Here's how the part is built. I have some questions about the finished solid (model axes, mm). A direction names the side the tool comes from. Round coordinates to 2 decimals unless told otherwise and drop trailing zeros. Loops run counter-clockwise (first coordinate to the right, second up) from the corner with the lowest first, then second, coordinate; pieces in that order, holes last. Notation, with made-up numbers: (15.25, 72) - (67.25, 72) arc R21 cw to (67.25, 98) - close; hole circle Ø2 at (37.5, -1.75). An arc over 180 degrees is marked (long way). Answer as a JSON object with one key per item and string values. Group by question number.
1) I want a section at C-C, the plane z = 0.3. Please give me the cut outline in (x, y), then the cut area to 3 significant figures.
2) If I drill on line 1 along X through (y, z) = (2.5, 1.2); line 2 along X through (y, z) = (-2, 2.1); line 3 along Z through (x, y) = (0, 3), over which ranges is the centre line in solid material (lowest first)? Write a range as [from, to].
3) Which directions (+Z, -Z, +X, -X, +Y, -Y) give clear straight access to the entire face, cutting with the end or side of a thin tool? Please do faces 1 (the face through (1.5, 0.6, 2)), 2 (the face through (-0.99, -4.42, 1.63)).
4) I want a section at B-B, the plane x = 1.75. Please give me the cut outline in (y, z).
5) Will these pins go through, and if not, where does the flat tip stop? P1, Ø2, axis at y = 4, z = 2, coming from the +X side; P2, Ø8, axis at x = 4, y = 5, coming from the +Z side; P3, Ø1.5, axis at x = -1.5, y = -4, coming from the +Z side; P4, Ø2, axis at x = 5.5, y = -3, coming from the +Z side.
6) If we mould it in two halves opening along Z, with no side actions, what happens to faces 3 (the face through (0, -2, 0)), 4 (the face through (7, 5, 2)), 5 (the face through (0.976, 5.054, 1.717))? For each: pulls with the +Z half, pulls with the -Z half, needs draft (parallel to the pull), parting line crosses it, or undercut.
7) I want a section at D-D, the plane x = 3.75. Please give me the cut outline in (y, z), then the cut area to 3 significant figures.
8) I want a section at A-A, the plane z = 1.45. Give the number of separate pieces and of enclosed holes in the cut face, then the cut area to 3 significant figures.
Autodesk Inventor part; units mm, degrees
ref_plane "YZ Plane" through (0, 0, 0) normal (1, 0, 0) x (0, 1, 0)
ref_plane "XZ Plane" through (0, 0, 0) normal (0, 1, 0) x (-1, 0, 0)
ref_plane "XY Plane" through (0, 0, 0) normal (0, 0, 1) x (1, 0, 0)
sketch "Base" plane through (0, 0, 0) normal (0, 0, 1) x (1, 0, 0)
  line L0 (-9, -3) -> (-9, 3)
  line L1 (-9, 3) -> (-4.5, 7.5)
  line L2 (-4.5, 7.5) -> (4.5, 7.5)
  line L3 (4.5, 7.5) -> (9, 3)
  line L4 (9, 3) -> (9, -3)
  line L5 (9, -3) -> (4.5, -7.5)
  line L6 (4.5, -7.5) -> (-4.5, -7.5)
  line L7 (-4.5, -7.5) -> (-9, -3)
  line L8 (-9, 0) -> (9, 0) construction
  line L9 (0, 7.5) -> (0, -7.5) construction
  point P0 (0, 0)
  point P1 (0, 0)
  dimension "d1" = 18
  dimension "d5" = 15
  dimension "d7" = 6
extrude "BaseFeature" add sketch "Base" along normal blind 4
fillet "BaseFilletsFeature" radius 3 8 edges at (-9, -3, 2) (-4.5, -7.5, 2) (4.5, -7.5, 2) (9, -3, 2) (9, 3, 2) (4.5, 7.5, 2) (-4.5, 7.5, 2) (-9, 3, 2)
sketch "RailHoles" plane through (0, 0, 4) normal (0, 0, 1) x (1, 0, 0)
  line L0 (2.1663, 4.1769) -> (5.6769, 0.6663) construction
  line L1 (-1.3568, 2.0431) -> (2.1538, -1.4675) construction
  line L2 (8.1213, 3.8787) -> (5.3787, 6.6213) construction
  line L3 (6.75, 5.25) -> (3.9216, 2.4216) construction
  circle A0 centre (2.1663, 4.1769) radius 1
  circle A1 centre (5.6769, 0.6663) radius 1
  circle A2 centre (-1.3568, 2.0431) radius 1
  circle A3 centre (2.1538, -1.4675) radius 1
  line L4 (2.8734, 4.884) -> (6.384, 1.3734)
  line L5 (1.4592, 3.4698) -> (4.9698, -0.0408)
  line L6 (-0.6497, 2.7502) -> (2.8609, -0.7604)
  line L7 (-2.0639, 1.336) -> (1.4467, -2.1746)
  dimension "d11" = 4
  dimension "d12" = 4
  dimension "d13" = 4.9647
  dimension "d14" = 2
  dimension "d15" = 1.5
  dimension "d25" = 3.8787
extrude "RailHolesFeature" cut sketch "RailHoles" against normal through all
sketch "RouteHole" plane through (-3.2574, -7.5, 0) normal (0, -1, 0) x (1, 0, 0)
  line L0 (6.5147, 4) -> (6.5147, 0) construction
  line L1 (0, 4) -> (6.5147, 4) construction
  line L2 (0, 0) -> (0, 4) construction
  line L3 (6.5147, 0) -> (0, 0) construction
  line L4 (0, 4) -> (0, 0) construction
  line L5 (0, 4) -> (6.5147, 4) construction
  line L6 (3.2574, 4) -> (3.2574, 0) construction
  line L7 (6.5147, 0) -> (0, 0) construction
  circle A0 centre (3.2574, 1.5) radius 1.25
  dimension "d40" = 2.5
  dimension "d41" = 1.5
hole "RouteHoleFeature" at (0, -7.5, 1.5) direction (0, 1, 0) diameter 2 end through all
sketch "SideProfile" plane through (9, -1.7574, 0) normal (1, 0, 0) x (0, 0, -1)
  arc A0 (-4, 9.2574) -> (-3, -5.7426) centre (109, 9.2574) ccw
  line L0 (-4, -5.7426) -> (0, -5.7426) construction
  line L1 (0, 9.2574) -> (-4, 9.2574) construction
  line L2 (-3, -5.7426) -> (0, -5.7426)
  line L3 (0, 9.2574) -> (0, -5.7426)
  line L4 (0, 9.2574) -> (0, 8.3787)
  line L5 (0, 9.2574) -> (-4, 9.2574)
  line L6 (-4, -2.1213) -> (-4, 0) construction
  dimension "d36" = 4
  dimension "d39" = 3
extrude "SideProfileFeature" cut sketch "SideProfile" against normal through all keep common part
equation "\"d7\" = 0.4 * d5"
equation "\"d12\" = 2 * d14"
equation "\"d13\" = 1.28 * d25"
properties part number "IndexRouter"
Outcome:
{
 "1": {"outline": "(-9, -1.76) arc R3 ccw to (-8.12, -3.88) - (-5.38, -6.62) arc R3 ccw to (-3.26, -7.5) - (3.26, -7.5) arc R3 ccw to (5.38, -6.62) - (8.12, -3.88) arc R3 ccw to (9, -1.76) - (9, 1.76) arc R3 ccw to (8.12, 3.88) - (5.38, 6.62) arc R3 ccw to (3.26, 7.5) - (-3.26, 7.5) arc R3 ccw to (-5.38, 6.62) - (-8.12, 3.88) arc R3 ccw to (-9, 1.76) - close; hole (-2.06, 1.34) - (1.45, -2.17) arc R1 ccw to (2.86, -0.76) - (-0.65, 2.75) arc R1 ccw to start; hole (1.46, 3.47) - (4.97, -0.04) arc R1 ccw to (6.38, 1.37) - (2.87, 4.88) arc R1 ccw to start", "area": "202 mm^2"},
 "2": {"line 1": "[-8.91, -2.25], [0.95, 2.43], [5.26, 8.91]", "line 2": "[-8.99, -0.8], [0.8, 1.27], [3, 8.99]", "line 3": "[0, 0.5], [2.5, 3.91]"},
 "3": {"face 1": "+Z, -Z", "face 2": "+Y, -Y"},
 "4": {"outline": "(-7.5, 0) - (-2.38, 0) - (-2.38, 3.57) arc R113 ccw to (-7.5, 3) - close; (0.35, 0) - (3.18, 0) - (3.18, 3.92) arc R113 ccw to (0.35, 3.77) - close; (5.09, 0) - (7.5, 0) - (7.5, 4) arc R113 ccw to (5.09, 3.97) - close"},
 "5": {"P1": "x = 8.73", "P2": "z = 4", "P3": "z = 3.49", "P4": "z = 3.6"},
 "6": {"face 3": "pulls with the -Z half", "face 4": "needs draft", "face 5": "undercut"},
 "7": {"outline": "(-7.46, 0) - (1.18, 0) - (1.18, 3.82) arc R113 ccw to (-7.46, 3.01) - close; (4.01, 0) - (7.46, 0) - (7.46, 4) arc R113 ccw to (4.01, 3.95) - close", "area": "43.7 mm^2"},
 "8": {"separate pieces": "2", "enclosed holes": "1", "area": "177 mm^2"}
}
